Answer from the drawing. Dimensions are ordinates in mm from the lowest x, y and z of the part. A direction names the side the tool comes from. Coordinates: 2 decimals unless noted, no trailing zeros. Order: outer loops, then holes, each group sorted by start corner. A loop starts at its lowest first (then second) coordinate and runs counter-clockwise, first axis right, second up. Notation, with made-up numbers: (75.25, 41) -> (102.25, 41) arc R11 cw to (102.25, 54) -> close; hole circle Ø5 at (14.25, 13.5). An arc over 180 degrees is marked (long way). Answer in a Markdown table with one row per item.
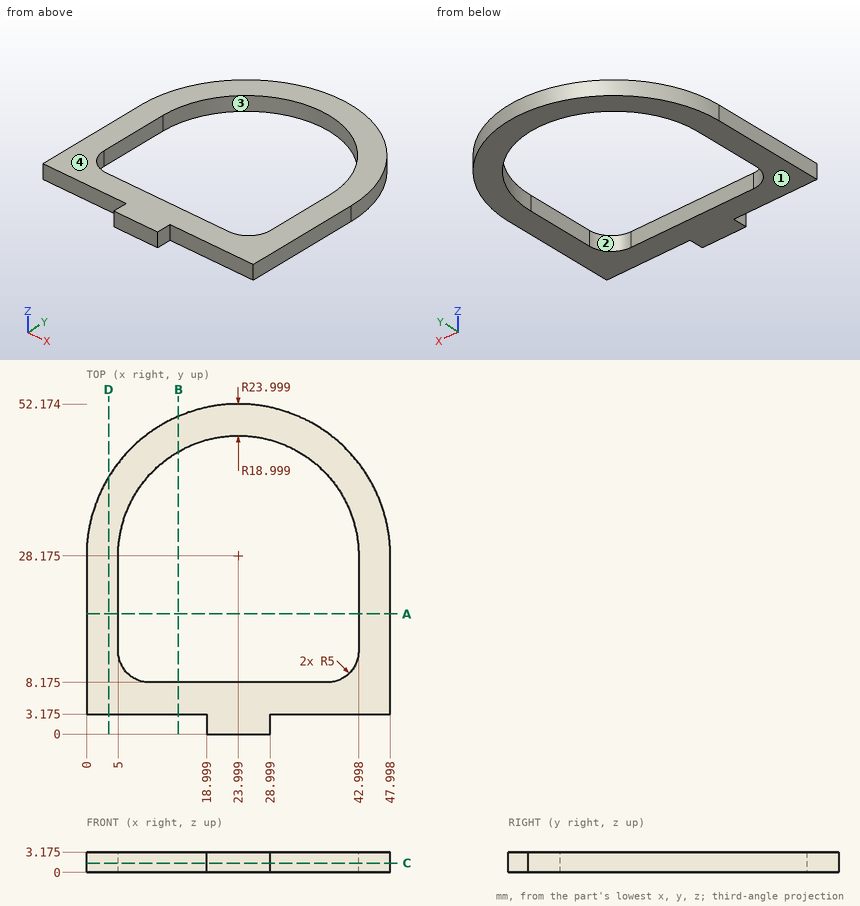
(1) Which of the six approach directions +Z, -Z, +X, -X, +Y, -Y give full straight-line access (tool end or side, diameter ignored) to the marked faces 3 and 4?
Check values:
| item | result |
|---|---|
| face 3 | +Z, -Z |
| face 4 | +Z, +X, -X, +Y, -Y |
(2) Flat-ended cylindrical pins translate along their axes: pin 1 (1 mm diameter, centred on x = 42, z = 1, fed in from -Y) (3 decimals); pin 2 (1 mm diameter, centred on x = 26, z = 1.5, fed in from +Y); pin 3 (1.6 mm diameter, centred on x = 24, z = 2, fed in from +Y). Find the tip coordinate at first contact, or state that the pin passes through.
Check values:
| item | result |
|---|---|
| pin 1 | y = 3.175 |
| pin 2 | y = 52.13 |
| pin 3 | y = 52.17 |
(3) Find the intervals of material crossed by line 1 along X through (y, z) = (18.5, 2.4); line 2 along Y through (x, z) = (17.5, 1.5) (1 decimal); line 3 along Y through (x, z) = (18.5, 1.6) (1 decimal), in increasing order. Write a range as from..to.
Check values:
| item | result |
|---|---|
| line 1 | 0..5, 43..48 |
| line 2 | 3.2..8.2, 46..51.3 |
| line 3 | 3.2..8.2, 46.4..51.5 |
(4) A cutting plane is placed at B-B, the plane x = 14.5. Determine the outline of the cut face in (y, z) (1 decimal).
Check values:
| item | result |
|---|---|
| outline | (3.2, 0) -> (8.2, 0) -> (8.2, 3.2) -> (3.2, 3.2) -> close; (44.6, 0) -> (50.2, 0) -> (50.2, 3.2) -> (44.6, 3.2) -> close |
(5) A cutting plane is placed at C-C, the plane z = 1.45. Determine the outline of the cut face in (x, y) (1 decimal).
Check values:
| item | result |
|---|---|
| outline | (0, 3.2) -> (19, 3.2) -> (19, 0) -> (29, 0) -> (29, 3.2) -> (48, 3.2) -> (48, 28.2) arc R24 ccw to (0, 28.2) -> close; hole (5, 13.2) arc R5 ccw to (10, 8.2) -> (38, 8.2) arc R5 ccw to (43, 13.2) -> (43, 28.2) arc R19 ccw to (5, 28.2) -> close |
(6) A cutting plane is placed at A-A, the plane y = 19. Determine the outline of the cut face in (x, z) (1 decimal).
Check values:
| item | result |
|---|---|
| outline | (0, 0) -> (5, 0) -> (5, 3.2) -> (0, 3.2) -> close; (43, 0) -> (48, 0) -> (48, 3.2) -> (43, 3.2) -> close |
(7) For a pull along Y with two mould halves and no side action, classify the marked faces 1 and 2 as released by +Y, released by -Y, zero draft, split by the parting line, or undercut.
Check values:
| item | result |
|---|---|
| face 1 | zero draft |
| face 2 | undercut |
(8) A cutting plane is placed at D-D, the plane x = 3.5. Determine the outline of the cut face in (y, z) (1 decimal), then the cut area to 3 significant figures.
Check values:
| item | result |
|---|---|
| outline | (3.2, 0) -> (40.7, 0) -> (40.7, 3.2) -> (3.2, 3.2) -> close |
| area | 119 mm² |
